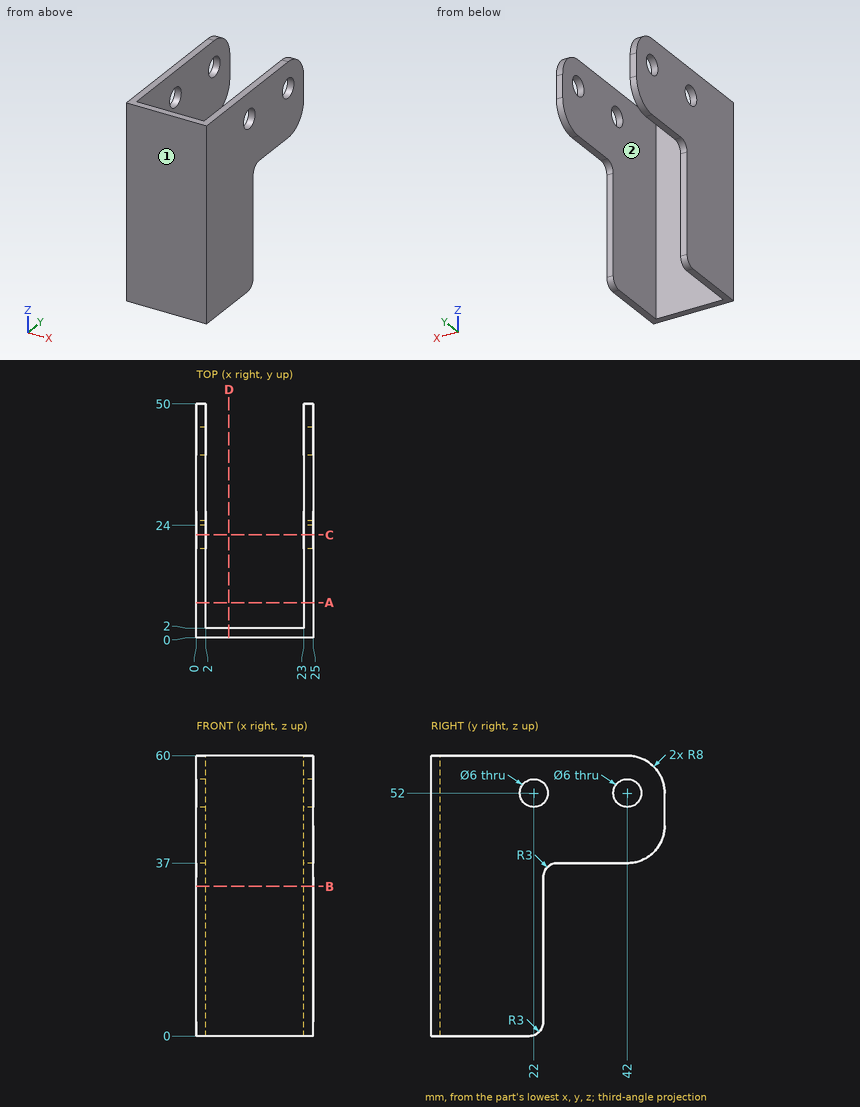
Can you work these out from the drawing? Everything is in mm from the part's minimum corner. A direction names the side the tool comes from. Give positions to 0.01 mm unless a question says otherwise; leave off trailing zeros. Loops run counter-clockwise (first coordinate to the right, second up) from the corner with the lowest first, then second, coordinate; pieces in that order, holes last. Notation, with made-up numbers: M -19.75,-14.75 L 10.25,-14.75 A6 cw 10.25,-4.75 Z; hole C 67.5,55.5 d4. An arc over 180 degrees is marked long. Put each result on its own line as item: value. Start each with the question number.
(1) I want a section at A-A on y = 7.5. Please give me the cut outline in (x, z), then the cut area to 3 significant figures.
(2) I need wall thicknesses on line 1 along Y through (x, z) = (1.55, 52); line 2 along X through (y, z) = (38.5, 53); line 3 along Z through (x, y) = (23.65, 22). Which ranges of each line are inside material? Lowest first, please. Write a range as [from, to].
(3) Will these pins go through, and if not, where does the flat tip stop? pin 1 Ø2 at (x, y) = (1.5, 34) entering from -Z; pin 2 Ø2 at (x, z) = (24, 22) entering from +Y; pin 3 Ø10.5 at (x, z) = (11, 34) entering from +Y.
(4) I want a section at B-B on z = 32. Please give me the cut outline in (x, y), then the cut area to 3 significant figures.
(5) For the marked faces 1 and 2, which set-ups out of +Z, -Z, +X, -X, +Y, -Y let a thin tool reach every point of the face, with its end or its side?
(6) I want a section at D-D on x = 7. Please give me the cut outline in (y, z), then the cut area to 3 significant figures.
(7) I want a section at C-C on y = 22. Please give me the cut outline in (x, z).
Answer block:
1. outline: M 0,0 L 2,0 L 2,60 L 0,60 Z; M 23,0 L 25,0 L 25,60 L 23,60 Z
1. area: 240 mm^2
2. line 1: [0, 19], [25, 39], [45, 50]
2. line 2: [0, 2], [23, 25]
2. line 3: [0.17, 49], [55, 60]
3. pin 1: z = 37
3. pin 2: y = 24
3. pin 3: y = 2
4. outline: M 0,0 L 25,0 L 25,24 L 23,24 L 23,2 L 2,2 L 2,24 L 0,24 Z
4. area: 138 mm^2
5. face 1: +Z, -Z, +X, -X, -Y
5. face 2: +Z, -Z, +Y
6. outline: M 0,0 L 2,0 L 2,60 L 0,60 Z
6. area: 120 mm^2
7. outline: M 0,0.17 L 2,0.17 L 2,49 L 0,49 Z; M 0,55 L 2,55 L 2,60 L 0,60 Z; M 23,0.17 L 25,0.17 L 25,49 L 23,49 Z; M 23,55 L 25,55 L 25,60 L 23,60 Z
